Here's how the part is built. I have some questions about the finished solid (model axes, mm). A direction names the side the tool comes from. Round coordinates to 2 decimals unless told otherwise and drop trailing zeros. Order: outer loops, then holes, each group sorted by start corner. A loop starts at its lowest first (then second) coordinate and runs counter-clockwise, first axis right, second up. Notation, with made-up numbers: (15, 65) -> (29, 65) arc R33 cw to (29, 96) -> close; hole circle Ø8 at (50, 0). An arc over 180 degrees is marked (long way). One line per item, written item: value.
```python
from build123d import *


with BuildPart() as part:
    # Sketch3 → Revolve1 (revolve)
    with BuildSketch(Plane.XY, mode=Mode.PRIVATE) as revolve1_sk:
        with BuildLine():
            Line((6.35, 12.95), (6.35, 5))
            Line((6.35, 5), (7.55, 5))
            Line((7.55, 5), (7.55, 14.15))
            Line((7.55, 14.15), (6.9, 14.15))
            Line((6.9, 14.15), (6.9, 19.3))
            Line((6.9, 19.3), (7.35, 19.3))
            Line((7.35, 19.3), (7.55, 19.5))
            Line((7.55, 19.5), (7.55, 28.622504621))
            ThreePointArc((7.55, 28.622504621), (7.449953131, 29.247146997), (7.159821902, 29.80929586))
            ThreePointArc((7.159821902, 29.80929586), (4.639195549, 34.693179743), (3.77, 40.12))
            Line((3.77, 40.12), (3.77, 43.62))
            Line((3.77, 43.62), (2.57, 43.62))
            Line((2.57, 43.62), (2.57, 40.12))
            Line((2.57, 40.12), (4.75, 29.3))
            Line((4.75, 29.3), (4.75, 20.5))
            Line((4.75, 20.5), (4.95, 20.5))
            Line((4.95, 20.5), (4.95, 12.95))
            Line((4.95, 12.95), (6.35, 12.95))
        make_face()
    revolve(revolve1_sk.sketch.rotate(Axis((0, 43.62, 0), (0, -1, 0)), 90), axis=Axis((0, 43.62, 0), (0, -1, 0)))


solid = part.part
```
Q1. For P1, Ø8, axis at y = 28, z = 2, coming from the -X side; P2, Ø4, axis at x = 0, z = 0, coming from the -Y side; P3, Ø6, axis at y = 21.5, z = -5, coming from the -X side; P4, Ø2, axis at x = 6, y = 19.5, coming from the -Z side, each with a flat end and sliding along its axis, tell me the tip position at first contact or that it passes through.
Answers:
P1: x = -7.55
P2: through
P3: x = -7.28
P4: z = -5.66
Q2. I want a section at A-A on y = 18.5. Write out the boundary of the cut face in (x, z), then the cut area to 3 significant figures.
Answers:
outline: circle Ø13.8 at (0, 0); hole circle Ø9.9 at (0, 0)
area: 72.6 mm2
Q3. If we mould it in two halves opening along X, with no side actions, what happens to faces 6 (the face through (2, 14.15, 7)), 7 (the face through (2.089, 35.836, -2.724)), 8 (the face through (7.37, 24.13, -1.64))? For each: pulls with the +X half, pulls with the -X half, needs draft (parallel to the pull), parting line crosses it, or undercut.
Answers:
face 6: needs draft
face 7: undercut
face 8: parting line crosses it
Q4. I need wall thicknesses on line 1 along X through (y, z) = (42.35, 0); line 2 along X through (y, z) = (8.25, 0); line 3 along Z through (x, y) = (-1.75, 20). Which ranges of each line are inside material? Lowest first, please.
Answers:
line 1: -3.77 to -2.57, 2.57 to 3.77
line 2: -7.55 to -6.35, 6.35 to 7.55
line 3: -7.34 to -4.63, 4.63 to 7.34
Q5. I want a section at B-B on y = 40.5. Write out the boundary of the cut face in (x, z), then the cut area to 3 significant figures.
Answers:
outline: circle Ø7.54 at (0, 0); hole circle Ø5.14 at (0, 0)
area: 23.9 mm2
Q6. Which directions (+Z, -Z, +X, -X, +Y, -Y) give clear straight access to the entire face, cutting with the end or side of a thin tool? Please do faces 1 (the face through (3.345, 41.894, 1.74)), 2 (the face through (2, 43.62, 2)), 3 (the face through (-4.66, 16.76, -5.09)), 4 (the face through (-2.55, 41.85, -0.33)), 5 (the face through (3.86, 8.92, -5.04)).
Answers:
face 1: +Y
face 2: +Z, -Z, +X, -X, +Y
face 3: none
face 4: +Y, -Y
face 5: -Y
